from build123d import *

# Parameters (mm, degrees)
CYLINDER204_R     = 2
CYLINDER204_DEPTH = 13
CYLINDER205_R     = 2
CYLINDER205_DEPTH = 13
CYLINDER203_R     = 2
CYLINDER203_DEPTH = 13
CYLINDER206_R     = 2
CYLINDER206_DEPTH = 13
BOX259_W          = 90
BOX259_H          = 100
BOX259_DEPTH      = 3


with BuildPart() as cylinder204:
    # Cylinder204 → Cylinder204 (new body)
    with BuildSketch(Plane(origin=(33, 55, 32), x_dir=(1, 0, 0), z_dir=(0, 0, 1))):
        Circle(CYLINDER204_R)
    extrude(amount=CYLINDER204_DEPTH)


with BuildPart() as cylinder205:
    # Cylinder205 → Cylinder205 (new body)
    with BuildSketch(Plane(origin=(-47, 55, 32), x_dir=(1, 0, 0), z_dir=(0, 0, 1))):
        Circle(CYLINDER205_R)
    extrude(amount=CYLINDER205_DEPTH)


with BuildPart() as cylinder203:
    # Cylinder203 → Cylinder203 (new body)
    with BuildSketch(Plane(origin=(33, -35, 32), x_dir=(1, 0, 0), z_dir=(0, 0, 1))):
        Circle(CYLINDER203_R)
    extrude(amount=CYLINDER203_DEPTH)


with BuildPart() as cylinder206:
    # Cylinder206 → Cylinder206 (new body)
    with BuildSketch(Plane(origin=(-47, -35, 32), x_dir=(1, 0, 0), z_dir=(0, 0, 1))):
        Circle(CYLINDER206_R)
    extrude(amount=CYLINDER206_DEPTH)


with BuildPart() as cut171:
    # Box259 → Box259 (new body)
    with BuildSketch(Plane(origin=(-52, -40, 42), x_dir=(1, 0, 0), z_dir=(0, 0, 1))):
        with Locations((45, 50)):
            Rectangle(BOX259_W, BOX259_H)
    extrude(amount=BOX259_DEPTH)

    # Cut168: cut Cylinder206
    add(cylinder206.part, mode=Mode.SUBTRACT)

    # Cut169: cut Cylinder203
    add(cylinder203.part, mode=Mode.SUBTRACT)

    # Cut170: cut Cylinder205
    add(cylinder205.part, mode=Mode.SUBTRACT)

    # Cut171: cut Cylinder204
    add(cylinder204.part, mode=Mode.SUBTRACT)


with BuildPart() as cut171_1:
    # Cut171 placement: moved
    add(cut171.part.moved(Location((0, 16, 15))))


solid = cut171_1.part
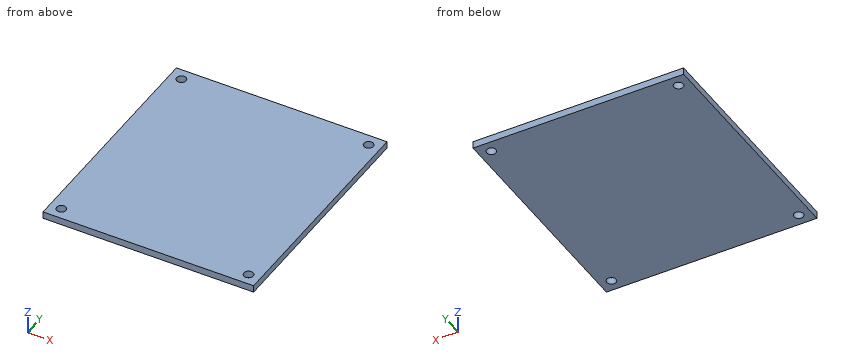
Work out the finished part from the listing and answer in its coordinate system (mm). Round coordinates to 2 decimals unless told otherwise and drop trailing zeros. Order: outer loops, then holes, each group sorted by start corner. A loop starts at its lowest first (then second) coordinate and runs counter-clockwise, first axis right, second up. Notation, with made-up numbers: M 66.5,72.25 L 86.5,72.25 A17 cw 86.5,94.25 Z; hole C 42.5,-22.5 d2. An arc over 180 degrees is marked long. Put each result on its own line as item: value. Start each with the question number.
Q1. Straight lines are drawn through the part: L1, parallel to X at y = -19, z = 57.9; L2, parallel to Y at x = 33, z = 58.45; L3, parallel to Y at x = -46, z = 59.25. For each, find the intervals that lie inside material, in ascending order. Write a range as [from, to].
Q2. Section B-B, the plane y = 71 is taken. Write down the section's boundary in (x, z), and give its area (3 significant figures).
Q3. A flat-ended cylindrical pin translates along its axis: pin 1 (3 mm diameter, centred on x = -47, y = 71, fed in from +Z). Find the tip coordinate at first contact, or state that the pin passes through.
Q4. Section A-A, the plane x = 33 is taken. Write down the section's boundary in (y, z), and give its area (3 significant figures).
Findings below:
1. L1: x = [-52, -49], [-45, 31], [35, 38]
1. L2: y = [-24, -21], [-17, 69], [73, 76]
1. L3: y = [-24, -20.73], [-17.27, 69.27], [72.73, 76]
2. outline: M -52,57 L -49,57 L -49,60 L -52,60 Z; M -45,57 L 31,57 L 31,60 L -45,60 Z; M 35,57 L 38,57 L 38,60 L 35,60 Z
2. area: 246 mm^2
3. pin 1: passes through
4. outline: M -24,57 L -21,57 L -21,60 L -24,60 Z; M -17,57 L 69,57 L 69,60 L -17,60 Z; M 73,57 L 76,57 L 76,60 L 73,60 Z
4. area: 276 mm^2
